For this review, use the dimensioned drawing (mm, ordinates from the lowest corner) and the shaded views. A direction names the side the tool comes from. Round coordinates to 2 decimals unless told otherwise and drop trailing zeros. Write each loop counter-clockwise with the first axis right and the second up, starting at its lowest first coordinate (ties: lowest second). Pieces come first, ordered by that corner, then holes. Notation, with made-up numbers: M -28,81 L 9,81 A13 ccw 9,101 Z; hole C -7,81 d10. An arc over 180 degrees is marked long. One line per question, with ' | ' between items. Start each with the question number.
Item 1: For L1, parallel to X at y = 8.75, z = 8 (1 decimal); L2, parallel to Z at x = 32, y = 23.25; L3, parallel to Z at x = 14.5, y = 10, list the stretches that pass through material, from the lowest coordinate up.
Item 2: Add section A-A, the plane z = 3.5. State the section outline as (x, y) points (1 decimal).
Item 3: Machinability: for the marked faces 5, 6 and 7, which of the approach directions +Z, -Z, +X, -X, +Y, -Y give a long, thin tool a straight path to every point of the face, cutting with its end or side? Answer none if there is none.
Item 4: Draft analysis for pull direction Y (two halves, no side actions). For the marked faces 1, 2, 3 and 4, state which applies: released by +Y, released by -Y, zero draft, split by the parting line, or undercut.
Item 5: Add section C-C, the plane x = 30.5. State the section outline as (y, z) points.
Item 6: Add section B-B, the plane y = 21.25. State the section outline as (x, z) points (1 decimal).
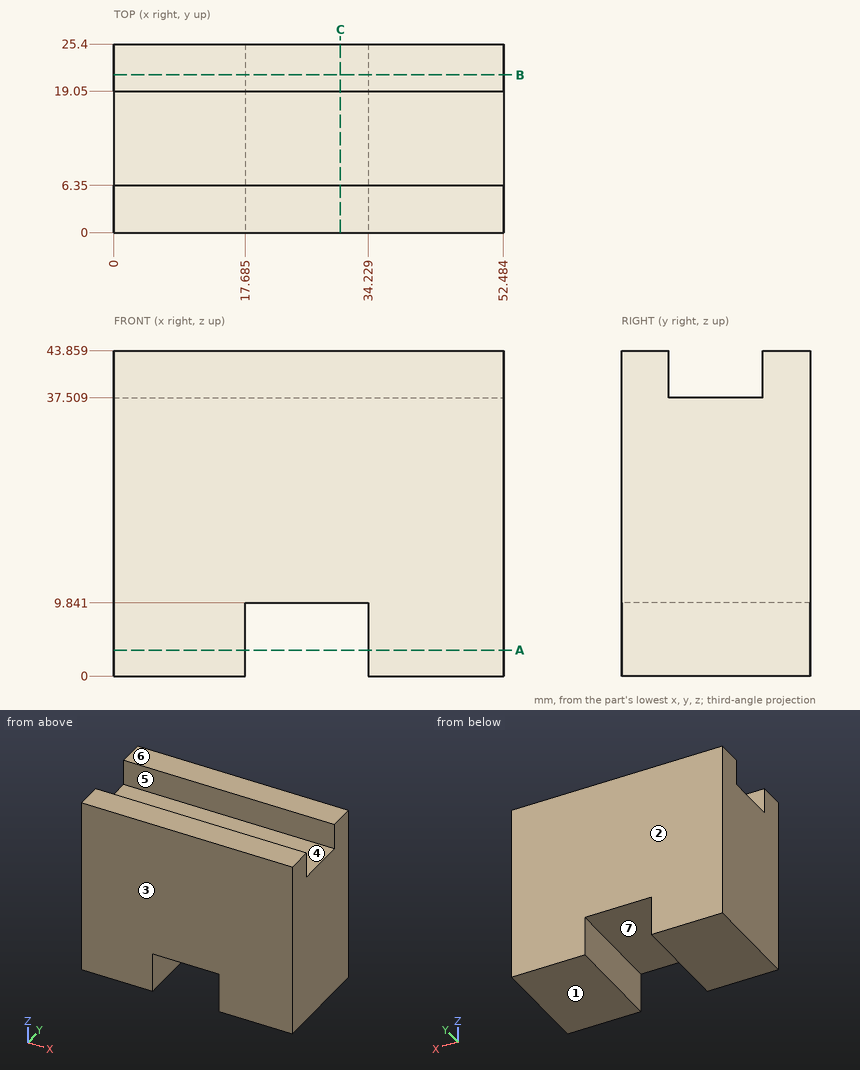
Computed values:
1) L1: x = 0 to 17.7, 34.2 to 52.5 | L2: z = 9.84 to 43.86 | L3: z = 0 to 37.51
2) outline: M 0,0 L 17.7,0 L 17.7,25.4 L 0,25.4 Z; M 34.2,0 L 52.5,0 L 52.5,25.4 L 34.2,25.4 Z
3) face 5: +Z, +X, -X | face 6: +Z, +X, -X, +Y, -Y | face 7: -Z, +Y, -Y
4) face 1: zero draft | face 2: released by +Y | face 3: released by -Y | face 4: undercut
5) outline: M 0,9.84 L 25.4,9.84 L 25.4,43.86 L 19.05,43.86 L 19.05,37.51 L 6.35,37.51 L 6.35,43.86 L 0,43.86 Z
6) outline: M 0,0 L 17.7,0 L 17.7,9.8 L 34.2,9.8 L 34.2,0 L 52.5,0 L 52.5,43.9 L 0,43.9 Z
